Work out the finished part from the listing and answer in its coordinate system (mm). Face numbers are marked on the shaded views. A direction names the side the tool comes from. Round coordinates to 2 decimals unless told otherwise and drop trailing zeros. Order: outer loops, then holes, each group sorted by start corner. A loop starts at its lowest first (then second) coordinate and runs counter-clockwise, first axis right, second up. Notation, with made-up numbers: M 82.25,79.5 L 119.25,79.5 A14 ccw 119.25,94.5 Z; hole C -11,18.25 d9. An arc over 180 degrees is marked long. Return JSON: item names as keys, results as strings.
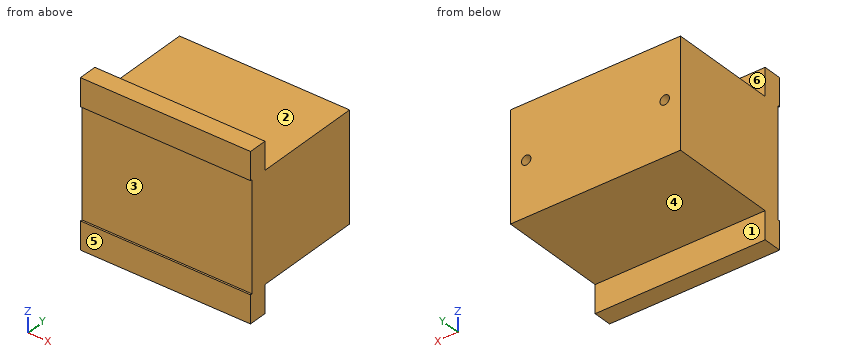
from build123d import *

# Parameters (mm, degrees)
SKETCH1_W                   = 92.1
SKETCH1_H                   = 88.7
BOSS_EXTRUDE1_DEPTH         = 10
SKETCH2_W                   = 92.1
SKETCH2_H                   = 58.7
BOSS_EXTRUDE2_DEPTH         = 58.8
SKETCH16_W                  = 92.1
SKETCH16_H                  = 58.7
CUT_EXTRUDE2_DEPTH          = 1
F_1_4_20_TAPPED_HOLE1_D     = 5.1054
F_1_4_20_TAPPED_HOLE1_DEPTH = 16.51
F_1_4_20_TAPPED_HOLE1_TIP   = 1.533816902


with BuildPart() as part:
    # Sketch1 → Boss-Extrude1 (new body)
    with BuildSketch(Plane(origin=(0, 0, 0), x_dir=(1, 0, 0), z_dir=(0, 1, 0))):
        Rectangle(SKETCH1_W, SKETCH1_H)
    extrude(amount=BOSS_EXTRUDE1_DEPTH)

    # Sketch2 → Boss-Extrude2 (add)
    with BuildSketch(Plane(origin=(0, 10, 0), x_dir=(1, 0, 0), z_dir=(0, 1, 0))):
        Rectangle(SKETCH2_W, SKETCH2_H)
    extrude(amount=BOSS_EXTRUDE2_DEPTH)

    # Sketch16 → Cut-Extrude2 (cut)
    with BuildSketch(Plane.XZ):
        Rectangle(SKETCH16_W, SKETCH16_H)
    extrude(amount=-CUT_EXTRUDE2_DEPTH, mode=Mode.SUBTRACT)

    # 1/4-20 Tapped Hole1
    with Locations(Plane(origin=(0, 68.8, 0), x_dir=(-1, 0, 0), z_dir=(0, 1, 0))):
        with Locations((37.5, 0), (-37.5, 0)):
            Hole(F_1_4_20_TAPPED_HOLE1_D / 2, depth=F_1_4_20_TAPPED_HOLE1_DEPTH)
            with Locations((0, 0, -(F_1_4_20_TAPPED_HOLE1_DEPTH + F_1_4_20_TAPPED_HOLE1_TIP / 2))):  # 118° drill point
                Cone(0, F_1_4_20_TAPPED_HOLE1_D / 2, F_1_4_20_TAPPED_HOLE1_TIP, mode=Mode.SUBTRACT)


solid = part.part
Item 1: The mould has two halves that part along Z. Classify the marked faces 1, 2 and 3: pulls with the +Z half, pulls with the -Z half, needs draft (parallel to the pull), parting line crosses it, or undercut.
Output:
{"face 1": "needs draft", "face 2": "pulls with the +Z half", "face 3": "undercut"}
Item 2: Find section A-A (x = -29). Determine the outline of the cut face in (y, z).
Output:
{"outline": "M 0,-44.35 L 10,-44.35 L 10,-29.35 L 68.8,-29.35 L 68.8,29.35 L 10,29.35 L 10,44.35 L 0,44.35 L 0,29.35 L 1,29.35 L 1,-29.35 L 0,-29.35 Z"}
Item 3: Find section C-C (y = 47). Determine the outline of the cut face in (x, z).
Output:
{"outline": "M -46.05,-29.35 L 46.05,-29.35 L 46.05,29.35 L -46.05,29.35 Z"}
Item 4: Consider line 1 along X through (y, z) = (62, 0); line 2 along Z through (x, y) = (-37.5, 63); line 3 along Y through (x, z) = (-13, 14.5). Determine where each line is inside the solid, lowest interval first. Write a range as [from, to].
Output:
{"line 1": "x = [-46.05, -40.05], [-34.95, 34.95], [40.05, 46.05]", "line 2": "z = [-29.35, -2.55], [2.55, 29.35]", "line 3": "y = [1, 68.8]"}
Item 5: Which of the six approach directions +Z, -Z, +X, -X, +Y, -Y give full straight-line access (tool end or side, diameter ignored) to the marked faces 4, 5 and 6?
Output:
{"face 4": "-Z, +X, -X, +Y", "face 5": "+Z, -Z, +X, -X, -Y", "face 6": "+Z, +X, -X, +Y"}
Item 6: Each of these flat-tipped pins is pushed along its axis until it touches: pin 1 (3 mm diameter, centred on x = 37.5, z = 0, fed in from -Y); pin 2 (1 mm diameter, centred on x = 14.5, y = 55.5, fed in from +Z); pin 3 (12 mm diameter, centred on x = -26, y = 44, fed in from -Z). Where does it stop, or does it pass through?
Output:
{"pin 1": "stops at y = 1", "pin 2": "stops at z = 29.35", "pin 3": "stops at z = -29.35"}
Item 7: Find section B-B (z = 31.5). Determine the outline of the cut face in (x, y), plus the area to 3 significant figures.
Output:
{"outline": "M -46.05,0 L 46.05,0 L 46.05,10 L -46.05,10 Z", "area": "921 mm^2"}
